```python
from build123d import *

# Parameters (mm, degrees)
SKETCH1_W      = 76.2
SKETCH1_H      = 3.175
HEAD_DEPTH     = 4.826
CHAMFER2_SIZE  = 0.635
CHAMFER2_SIZE2 = 0.6351
FILLET_2_R     = 0.635


with BuildPart() as part:
    # Sketch1 → Body (revolve)
    with BuildSketch(Plane.XY):
        with Locations((38.1, 1.5875)):
            Rectangle(SKETCH1_W, SKETCH1_H)
    revolve(axis=Axis((76.2, 0, 0), (-1, 0, 0)))

    # Sketch2 → Head (add)
    with BuildSketch(Plane.ZY):
        Polygon((0, 5.499261314), (4.7625, 2.749630657), (4.7625, -2.749630657), (0, -5.499261314), (-4.7625, -2.749630657), (-4.7625, 2.749630657), align=None)
    extrude(amount=HEAD_DEPTH)

    # Sketch3 → Thread (revolve, cut)
    with BuildSketch(Plane.XY):
        Polygon((-4.826, 4.7625), (-4.276073869, 5.715), (-4.826, 5.715), align=None)
    revolve(axis=Axis((-1.1, 0, 0), (1, 0, 0)), mode=Mode.SUBTRACT)

    # Chamfer2
    chamfer2_edges = [part.edges().sort_by_distance(p)[0] for p in [
        (76.2, -3.175, 0),
    ]]
    chamfer2_side = [part.faces().sort_by_distance(p)[0] for p in [
        (38.1, -3.175, 0),
    ]]
    chamfer(chamfer2_edges, length=CHAMFER2_SIZE, length2=CHAMFER2_SIZE2, reference=chamfer2_side[0])

    # Fillet 2
    fillet_2_edges = [part.edges().sort_by_distance(p)[0] for p in [
        (0, -3.175, 0),
    ]]
    fillet(fillet_2_edges, radius=FILLET_2_R)


solid = part.part
```
Work out the finished part from the listing and answer in its coordinate system (mm). A direction names the side the tool comes from. Coordinates: 2 decimals unless noted, no trailing zeros. Loops run counter-clockwise (first coordinate to the right, second up) from the corner with the lowest first, then second, coordinate; pieces in that order, holes last.
1) Flat-ended cylindrical pins translate along their axes: pin 1 (1 mm diameter, centred on x = 18.5, z = 1.5, fed in from -Y); pin 2 (5 mm diameter, centred on x = 15, y = 2, fed in from +Z) (3 decimals). Find the tip coordinate at first contact, or state that the pin passes through.
Results:
pin 1: stops at y = -3.01
pin 2: stops at z = 3.175
2) Section A-A (x = 50) is taken. Give the vertices of the cut face in (y, z) (3 decimals).
Results:
outline: circle Ø6.35 at (0, 0)
3) Consider probe 1 along X at (y, z) = (-0.25, -4); probe 2 along Y at (x, z) = (33, 0) (3 decimals); probe 3 along Y at (x, z) = (56.5, -0.75). Determine where each line is inside the solid, lowest interval first.
Results:
probe 1: x = -4.83 to 0
probe 2: y = -3.175 to 3.175
probe 3: y = -3.09 to 3.09
4) For faces 1 (the conical face through (-4.72, -2.46, 4.29)), 2 (the cylindrical face through (38.62, -0.69, 3.1)), determine the directions among +Z, -Z, +X, -X, +Y, -Y from which every point of the face is accessible in a straight line to the end or side of a thin tool.
Results:
face 1: +Z, -X, -Y
face 2: +X
